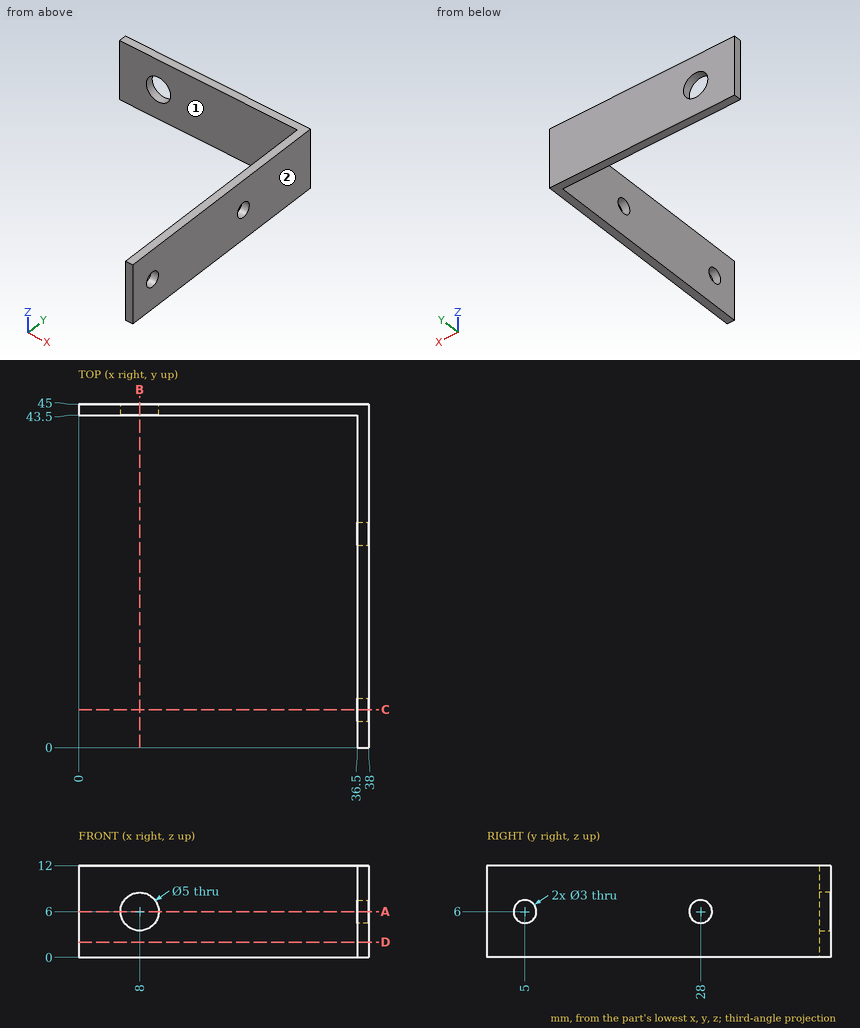
The figure shows three views and two pictorial views of one solid part (mm, origin at its lowest corner). Answer the questions. A direction names the side the tool comes from. Give positions to 0.01 mm unless a question says otherwise; leave off trailing zeros. Write each loop counter-clockwise with the first axis right and the second up, starting at its lowest first coordinate (ties: lowest second). Pieces come first, ordered by that corner, then holes. Notation, with made-up numbers: (38, 48.25) -> (71, 48.25) arc R11 cw to (71, 55.25) -> close; hole circle Ø7 at (6, 21). An arc over 180 degrees is marked (long way). Use one line per item in the form item = value.
1) Section A-A on z = 6 is taken. Write down the section's boundary in (x, y), plus the area to 3 significant figures.
Result:
outline = (0, 43.5) -> (5.5, 43.5) -> (5.5, 45) -> (0, 45) -> close; (10.5, 43.5) -> (36.5, 43.5) -> (36.5, 29.5) -> (38, 29.5) -> (38, 45) -> (10.5, 45) -> close; (36.5, 0) -> (38, 0) -> (38, 3.5) -> (36.5, 3.5) -> close; (36.5, 6.5) -> (38, 6.5) -> (38, 26.5) -> (36.5, 26.5) -> close
area = 106 mm²
2) Section B-B on x = 8 is taken. Write down the section's boundary in (y, z), plus the area to 3 significant figures.
Result:
outline = (43.5, 0) -> (45, 0) -> (45, 3.5) -> (43.5, 3.5) -> close; (43.5, 8.5) -> (45, 8.5) -> (45, 12) -> (43.5, 12) -> close
area = 10.5 mm²
3) Straight lines are drawn through the part: probe 1 along Y at (x, z) = (37.3, 6); probe 2 along X at (y, z) = (44, 6); probe 3 along X at (y, z) = (26.5, 0.5). For each, find the intervals that lie inside material, in ascending order.
Result:
probe_1 = 0 to 3.5, 6.5 to 26.5, 29.5 to 45
probe_2 = 0 to 5.5, 10.5 to 38
probe_3 = 36.5 to 38
4) Section D-D on z = 2 is taken. Write down the section's boundary in (x, y), plus the area to 3 significant figures.
Result:
outline = (0, 43.5) -> (36.5, 43.5) -> (36.5, 0) -> (38, 0) -> (38, 45) -> (0, 45) -> close
area = 122 mm²
5) Section C-C on y = 5 is taken. Write down the section's boundary in (x, z), plus the area to 3 significant figures.
Result:
outline = (36.5, 0) -> (38, 0) -> (38, 4.5) -> (36.5, 4.5) -> close; (36.5, 7.5) -> (38, 7.5) -> (38, 12) -> (36.5, 12) -> close
area = 13.5 mm²
6) Each of these flat-tipped pins is pushed along its axis until it touches: P1, Ø4, axis at y = 36, z = 8.5, coming from the -X side; P2, Ø3.5, axis at x = 9, z = 4.5, coming from the -Y side. Where does it stop, or does it pass through?
Result:
P1 = 36.5
P2 = 43.5
7) A tool of negligible diameter and unlimited length cuts with its end or side. For the marked faces 1 and 2, from which of +Z, -Z, +X, -X, +Y, -Y can it reach the whole face along a straight path? Write none if from no direction.
Result:
face_1 = +Z, -Z, -X, -Y
face_2 = +Z, -Z, +X, +Y, -Y
